Verification items for the finished model (mm, model axes). Face numbers are marked on the shaded views. Coordinates: 2 decimals unless noted, no trailing zeros. Write each loop counter-clockwise with the first axis right and the second up, starting at its lowest first coordinate (ties: lowest second). Pieces come first, ordered by that corner, then holes. Notation, with made-up numbers: (23, 10) - (69, 10) arc R17 ccw to (69, 18) - close; hole circle Ø9 at (-7, 32). An arc over 180 degrees is marked (long way). Use one line per item in the form item = value. Start each with the question number.
(1) Material ranges on line 1 (X direction, y = 98, z = 9.5); line 2 (Y direction, x = 98, z = 50.5); line 3 (Y direction, x = 7, z = 53.5), recorded low to high. Write a range as [from, to].
(2) Sectioned sample at B-B (y = 67.5). Record the cut outline in (x, z).
(3) Sectioned sample at C-C (z = 46.5). Count the separate pieces of the cut face and the enclosed holes in it, and give its area (3 significant figures).
(4) Sectioned sample at D-D (y = 88.5). Record the cut outline in (x, z), and give its area (3 significant figures).
(5) Mould release check, pull along X, two halves, no side actions. Record for the marked faces 1, 2 and 3: released by +X, released by -X, zero draft, split by the parting line, or undercut.
(6) Sectioned sample at A-A (x = 160). Record the cut outline in (y, z).
(7) Gauge pin test, flat ends, axial feed: pin 1 Ø3 at (x, y) = (41, 96.5) entering from +Z; pin 2 Ø20 at (x, y) = (139, 144) entering from +Z; pin 3 Ø1 at (x, y) = (26, 130.5) entering from +Z. Record the tip position at first contact, or that the pin passes through.
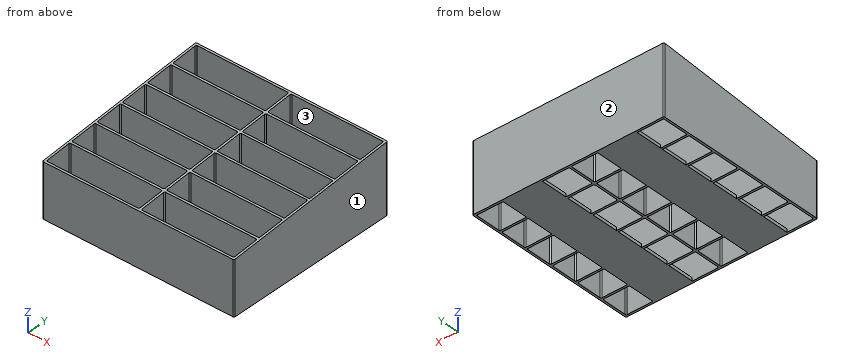
from build123d import *

# Parameters (mm, degrees)
PAD_DEPTH    = 65
POCKET_DEPTH = 180.001
SKETCH002_W  = 37
SKETCH002_H  = 164
PAD001_DEPTH = 3


with BuildPart() as part:
    # Sketch → Pad (new body)
    with BuildSketch(Plane.XY):
        with BuildLine():
            ThreePointArc((1, 164), (0.292893, 163.707107), (0, 163))
            Line((0, 1), (0, 163))
            ThreePointArc((0, 1), (0.292893, 0.292893), (1, 0))
            Line((179, 0), (1, 0))
            ThreePointArc((179, 0), (179.707107, 0.292893), (180, 1))
            Line((180, 1), (180, 163))
            ThreePointArc((180, 163), (179.707107, 163.707107), (179, 164))
            Line((179, 164), (1, 164))
        make_face()
        with BuildLine():
            ThreePointArc((3, 27), (2.292893, 26.707107), (2, 26))
            Line((2, 3), (2, 26))
            ThreePointArc((2, 3), (2.292893, 2.292893), (3, 2))
            Line((3, 2), (88, 2))
            ThreePointArc((88, 2), (88.707107, 2.292893), (89, 3))
            Line((89, 3), (89, 26))
            ThreePointArc((89, 26), (88.707107, 26.707107), (88, 27))
            Line((3, 27), (88, 27))
        make_face(mode=Mode.SUBTRACT)
        with BuildLine():
            ThreePointArc((2, 30), (2.292893, 29.292893), (3, 29))
            Line((3, 29), (88, 29))
            ThreePointArc((88, 29), (88.707107, 29.292893), (89, 30))
            Line((89, 53), (89, 30))
            ThreePointArc((89, 53), (88.707107, 53.707107), (88, 54))
            Line((3, 54), (88, 54))
            ThreePointArc((3, 54), (2.292893, 53.707107), (2, 53))
            Line((2, 53), (2, 30))
        make_face(mode=Mode.SUBTRACT)
        with BuildLine():
            ThreePointArc((2, 84), (2.292893, 83.292893), (3, 83))
            Line((3, 83), (88, 83))
            ThreePointArc((88, 83), (88.707107, 83.292893), (89, 84))
            Line((89, 107), (89, 84))
            ThreePointArc((89, 107), (88.707107, 107.707107), (88, 108))
            Line((3, 108), (88, 108))
            ThreePointArc((3, 108), (2.292893, 107.707107), (2, 107))
            Line((2, 107), (2, 84))
        make_face(mode=Mode.SUBTRACT)
        with BuildLine():
            ThreePointArc((3, 81), (2.292893, 80.707107), (2, 80))
            Line((2, 57), (2, 80))
            ThreePointArc((2, 57), (2.292893, 56.292893), (3, 56))
            Line((3, 56), (88, 56))
            ThreePointArc((88, 56), (88.707107, 56.292893), (89, 57))
            Line((89, 57), (89, 80))
            ThreePointArc((89, 80), (88.707107, 80.707107), (88, 81))
            Line((3, 81), (88, 81))
        make_face(mode=Mode.SUBTRACT)
        with BuildLine():
            ThreePointArc((3, 135), (2.292893, 134.707107), (2, 134))
            Line((2, 111), (2, 134))
            ThreePointArc((2, 111), (2.292893, 110.292893), (3, 110))
            Line((3, 110), (88, 110))
            ThreePointArc((88, 110), (88.707107, 110.292893), (89, 111))
            Line((89, 111), (89, 134))
            ThreePointArc((89, 134), (88.707107, 134.707107), (88, 135))
            Line((3, 135), (88, 135))
        make_face(mode=Mode.SUBTRACT)
        with BuildLine():
            ThreePointArc((2, 138), (2.292893, 137.292893), (3, 137))
            Line((3, 137), (88, 137))
            ThreePointArc((88, 137), (88.707107, 137.292893), (89, 138))
            Line((89, 161), (89, 138))
            ThreePointArc((89, 161), (88.707107, 161.707107), (88, 162))
            Line((3, 162), (88, 162))
            ThreePointArc((3, 162), (2.292893, 161.707107), (2, 161))
            Line((2, 161), (2, 138))
        make_face(mode=Mode.SUBTRACT)
        with BuildLine():
            ThreePointArc((178, 26), (177.707107, 26.707107), (177, 27))
            Line((177, 27), (92, 27))
            ThreePointArc((92, 27), (91.292893, 26.707107), (91, 26))
            Line((91, 3), (91, 26))
            ThreePointArc((91, 3), (91.292893, 2.292893), (92, 2))
            Line((177, 2), (92, 2))
            ThreePointArc((177, 2), (177.707107, 2.292893), (178, 3))
            Line((178, 3), (178, 26))
        make_face(mode=Mode.SUBTRACT)
        with BuildLine():
            ThreePointArc((177, 29), (177.707107, 29.292893), (178, 30))
            Line((178, 53), (178, 30))
            ThreePointArc((178, 53), (177.707107, 53.707107), (177, 54))
            Line((177, 54), (92, 54))
            ThreePointArc((92, 54), (91.292893, 53.707107), (91, 53))
            Line((91, 53), (91, 30))
            ThreePointArc((91, 30), (91.292893, 29.292893), (92, 29))
            Line((177, 29), (92, 29))
        make_face(mode=Mode.SUBTRACT)
        with BuildLine():
            ThreePointArc((177, 83), (177.707107, 83.292893), (178, 84))
            Line((178, 107), (178, 84))
            ThreePointArc((178, 107), (177.707107, 107.707107), (177, 108))
            Line((177, 108), (92, 108))
            ThreePointArc((92, 108), (91.292893, 107.707107), (91, 107))
            Line((91, 107), (91, 84))
            ThreePointArc((91, 84), (91.292893, 83.292893), (92, 83))
            Line((177, 83), (92, 83))
        make_face(mode=Mode.SUBTRACT)
        with BuildLine():
            ThreePointArc((178, 80), (177.707107, 80.707107), (177, 81))
            Line((177, 81), (92, 81))
            ThreePointArc((92, 81), (91.292893, 80.707107), (91, 80))
            Line((91, 57), (91, 80))
            ThreePointArc((91, 57), (91.292893, 56.292893), (92, 56))
            Line((177, 56), (92, 56))
            ThreePointArc((177, 56), (177.707107, 56.292893), (178, 57))
            Line((178, 57), (178, 80))
        make_face(mode=Mode.SUBTRACT)
        with BuildLine():
            ThreePointArc((178, 134), (177.707107, 134.707107), (177, 135))
            Line((177, 135), (92, 135))
            ThreePointArc((92, 135), (91.292893, 134.707107), (91, 134))
            Line((91, 111), (91, 134))
            ThreePointArc((91, 111), (91.292893, 110.292893), (92, 110))
            Line((177, 110), (92, 110))
            ThreePointArc((177, 110), (177.707107, 110.292893), (178, 111))
            Line((178, 111), (178, 134))
        make_face(mode=Mode.SUBTRACT)
        with BuildLine():
            ThreePointArc((177, 137), (177.707107, 137.292893), (178, 138))
            Line((178, 161), (178, 138))
            ThreePointArc((178, 161), (177.707107, 161.707107), (177, 162))
            Line((177, 162), (92, 162))
            ThreePointArc((92, 162), (91.292893, 161.707107), (91, 161))
            Line((91, 161), (91, 138))
            ThreePointArc((91, 138), (91.292893, 137.292893), (92, 137))
            Line((177, 137), (92, 137))
        make_face(mode=Mode.SUBTRACT)
    extrude(amount=PAD_DEPTH)

    # Sketch001 (on Face2 of Pad) → Pocket (cut, through all)
    with BuildSketch(Plane.YZ.offset(180)):
        Polygon((0, 50), (202.776713, 67.740664), (191.336548, 87.155762), (-16.35232, 87.155762), align=None)
    extrude(amount=-POCKET_DEPTH, mode=Mode.SUBTRACT)

    # Sketch002 (on Face2 of Pocket) → Pad001 (join)
    with BuildSketch(Plane(origin=(0, 0, 0), x_dir=(1, 0, 0), z_dir=(0, 0, -1))):
        with Locations((45.5, -82)):
            Rectangle(SKETCH002_W, SKETCH002_H)
        with Locations((134.5, -82)):
            Rectangle(SKETCH002_W, SKETCH002_H)
    extrude(amount=-PAD001_DEPTH)


solid = part.part
Answers below:
q1.line_1 = [0, 2], [89, 91], [178, 180]
q1.line_2 = [27, 29], [54, 56], [81, 83], [108, 110], [135, 137], [162, 164]
q1.line_3 = [54, 56], [81, 83], [108, 110], [135, 137], [162, 164]
q2.outline = (0, 0) - (2, 0) - (2, 55.91) - (0, 55.91) - close; (27, 0) - (64, 0) - (64, 3) - (27, 3) - close; (89, 0) - (91, 0) - (91, 55.91) - (89, 55.91) - close; (116, 0) - (153, 0) - (153, 3) - (116, 3) - close; (178, 0) - (180, 0) - (180, 55.91) - (178, 55.91) - close
q3.separate_pieces = 1
q3.enclosed_holes = 12
q3.area = 3,430 mm2
q4.outline = (0, 0) - (2, 0) - (2, 57.74) - (0, 57.74) - close; (27, 0) - (64, 0) - (64, 3) - (27, 3) - close; (89, 0) - (91, 0) - (91, 57.74) - (89, 57.74) - close; (116, 0) - (153, 0) - (153, 3) - (116, 3) - close; (178, 0) - (180, 0) - (180, 57.74) - (178, 57.74) - close
q4.area = 568 mm2
q5.face_1 = released by +X
q5.face_2 = zero draft
q5.face_3 = undercut
q6.outline = (0, 0) - (2, 0) - (2, 50.17) - (0, 50) - close; (27, 0) - (29, 0) - (29, 52.54) - (27, 52.36) - close; (54, 0) - (56, 0) - (56, 54.9) - (54, 54.72) - close; (81, 0) - (83, 0) - (83, 57.26) - (81, 57.09) - close; (108, 0) - (110, 0) - (110, 59.62) - (108, 59.45) - close; (135, 0) - (137, 0) - (137, 61.99) - (135, 61.81) - close; (162, 0) - (164, 0) - (164, 64.35) - (162, 64.17) - close
q7.pin_1 = 3
q7.pin_2 = 61.99
q7.pin_3 = through
